Part model, mm, in its own coordinate system. Face numbers are marked on the shaded views. Round coordinates to 2 decimals unless told otherwise and drop trailing zeros. Loops run counter-clockwise (first coordinate to the right, second up) from the corner with the lowest first, then second, coordinate; pieces in that order, holes last. Notation, with made-up numbers: M 6,-21.5 L 26,-21.5 A20 ccw 26,2.5 Z; hole C 3,11 d6. An arc over 180 degrees is marked long. Write each question's results on one line, items separated by ' | '.
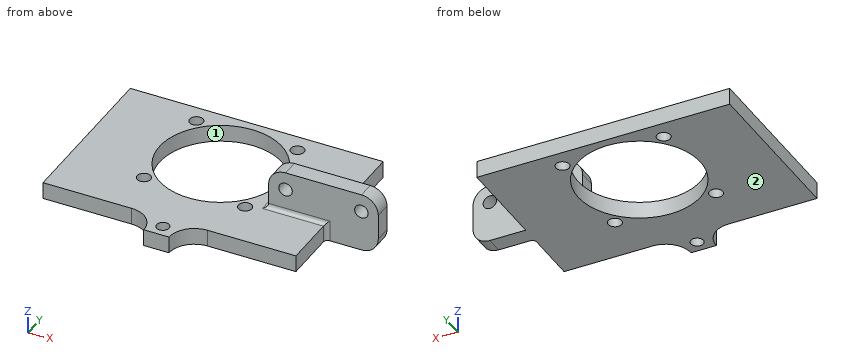
from build123d import *

# Parameters (mm, degrees)
SKETCH1_W                = 60
SKETCH1_H                = 40
BOSS_EXTRUDE1_DEPTH      = 4
SKETCH4_R                = 14.5
CUT_EXTRUDE1_DEPTH       = 4
SKETCH6_R                = 1.6
CUT_EXTRUDE2_DEPTH       = 4
SKETCH7_W                = 26
SKETCH7_H                = 4
BOSS_EXTRUDE3_DEPTH      = 10
SKETCH8_R                = 1.6
CUT_EXTRUDE3_DEPTH       = 78.162231694
SKETCH9_W                = 4
SKETCH9_H                = 4
BOSS_EXTRUDE4_DEPTH      = 12.5
FILLET2_R                = 4
FILLET3_R                = 1
SKETCH10_W               = 6
SKETCH10_H               = 4
BOSS_EXTRUDE5_DEPTH      = 6
FILLET4_R                = 6
F_3_0_3_DIAMETER_HOLE1_D = 3


with BuildPart() as part:
    # Sketch1 → Boss-Extrude1 (new body)
    with BuildSketch(Plane.XY):
        with Locations((30, 20)):
            Rectangle(SKETCH1_W, SKETCH1_H)
    extrude(amount=BOSS_EXTRUDE1_DEPTH)

    # Sketch4 → Cut-Extrude1 (cut)
    with BuildSketch(Plane.XY.offset(4)):
        with Locations((30, 23.5)):
            Circle(SKETCH4_R)
    extrude(amount=-CUT_EXTRUDE1_DEPTH, mode=Mode.SUBTRACT)

    # Sketch6 → Cut-Extrude2 (cut)
    with BuildSketch(Plane.XY.offset(4)):
        with Locations((42, 11.5)):
            Circle(SKETCH6_R)
        with Locations((18, 11.5)):
            Circle(SKETCH6_R)
        with Locations((18, 35.5)):
            Circle(SKETCH6_R)
        with Locations((42, 35.5)):
            Circle(SKETCH6_R)
    extrude(amount=-CUT_EXTRUDE2_DEPTH, mode=Mode.SUBTRACT)

    # Sketch7 → Boss-Extrude3 (add)
    with BuildSketch(Plane.XY.offset(4)):
        with Locations((59.5, 15.6)):
            Rectangle(SKETCH7_W, SKETCH7_H)
    extrude(amount=BOSS_EXTRUDE3_DEPTH)

    # Sketch8 → Cut-Extrude3 (cut, through all)
    with BuildSketch(Plane(origin=(0, 17.6, 0), x_dir=(1, 0, 0), z_dir=(0, 1, 0))):
        with Locations(Location((68.5, -9.75, 0), (0, 0, 270))):
            Circle(SKETCH8_R)
        with Locations(Location((50.5, -9.75, 0), (0, 0, 270))):
            Circle(SKETCH8_R)
    extrude(amount=-CUT_EXTRUDE3_DEPTH, mode=Mode.SUBTRACT)

    # Sketch9 → Boss-Extrude4 (add)
    with BuildSketch(Plane(origin=(60, 0, 0), x_dir=(0, 0, -1), z_dir=(1, 0, 0))):
        with Locations((-2, 15.6)):
            Rectangle(SKETCH9_W, SKETCH9_H)
    extrude(amount=BOSS_EXTRUDE4_DEPTH)

    # Fillet2
    fillet2_edges = [part.edges().sort_by_distance(p)[0] for p in [
        (46.5, 15.6, 14),
        (72.5, 15.6, 14),
        (72.5, 15.6, 0),
    ]]
    fillet(fillet2_edges, radius=FILLET2_R)

    # Fillet3
    fillet3_edges = [part.edges().sort_by_distance(p)[0] for p in [
        (46.5, 15.6, 4),
        (53.25, 13.6, 4),
        (60, 13.6, 2),
    ]]
    fillet(fillet3_edges, radius=FILLET3_R)

    # Sketch10 → Boss-Extrude5 (add)
    with BuildSketch(Plane.XZ):
        with Locations((30, 2)):
            Rectangle(SKETCH10_W, SKETCH10_H)
    extrude(amount=BOSS_EXTRUDE5_DEPTH)

    # Fillet4
    fillet4_edges = [part.edges().sort_by_distance(p)[0] for p in [
        (27, 0, 2),
        (33, 0, 2),
    ]]
    fillet(fillet4_edges, radius=FILLET4_R - 0.0001)  # a hair under: the kernel refuses the full size

    # Ø3.0 (3) Diameter Hole1 (through all)
    with Locations(Plane.XY.offset(4)):
        with Locations((30, -3)):
            Hole(F_3_0_3_DIAMETER_HOLE1_D / 2)


solid = part.part
Item 1: Band-saw the part on B-B on x = 18. Give the cut face in (y, z).
Filled sheet:
outline: M 0,0 L 9.9,0 L 9.9,4 L 0,4 Z; M 13.1,0 L 15.36,0 L 15.36,4 L 13.1,4 Z; M 31.64,0 L 33.9,0 L 33.9,4 L 31.64,4 Z; M 37.1,0 L 40,0 L 40,4 L 37.1,4 Z
Item 2: Band-saw the part on A-A on y = 23.5. Give the cut face in (x, z), and give its area (3 significant figures).
Filled sheet:
outline: M 0,0 L 15.5,0 L 15.5,4 L 0,4 Z; M 44.5,0 L 60,0 L 60,4 L 44.5,4 Z | area: 124 mm^2
Item 3: Drop flat-ended pins along their axis: P1, Ø4.5, axis at x = 50, z = 2.5, coming from the -Y side; P2, Ø4.5, axis at y = 16.5, z = 7.5, coming from the -X side; P3, Ø1, axis at y = 7, z = 3.5, coming from the +X side. Give the stop position or say it passes through.
Filled sheet:
P1: y = 0 | P2: x = 46.5 | P3: x = 60
Item 4: Two-plate mould, pull along X, no slides. Class the marked faces 1 and 2: +X half, -X half, draft (parallel to the pull), parting line (faces both ways), or undercut.
Filled sheet:
face 1: undercut | face 2: draft
Item 5: Band-saw the part on C-C on x = 37.5. Give the cut face in (y, z).
Filled sheet:
outline: M -0.19,0 L 11.09,0 L 11.09,4 L -0.19,4 Z; M 35.91,0 L 40,0 L 40,4 L 35.91,4 Z
Item 6: Wall check: L1, parallel to Y at x = 30, z = 2.75; L2, parallel to X at y = 14.85, z = 9.75; L3, parallel to Z at x = 68.5, y = 14.9. Give the ranges that are in metal, low to high.
Filled sheet:
L1: -6 to -4.5, -1.5 to 9, 38 to 40 | L2: 46.5 to 48.9, 52.1 to 66.9, 70.1 to 72.5 | L3: 0 to 8.15, 11.35 to 14
Item 7: Band-saw the part on D-D on z = 1.5. Count the separate pieces of the cut face and the enclosed holes in it, and give its area (3 significant figures).
Filled sheet:
separate pieces: 1 | enclosed holes: 6 | area: 1,800 mm^2
